Part model, mm, in its own coordinate system. Coordinates: 2 decimals unless noted, no trailing zeros. Loops run counter-clockwise (first coordinate to the right, second up) from the corner with the lowest first, then second, coordinate; pieces in that order, holes last. Notation, with made-up numbers: (-13.5, 50) - (-1.5, 50) arc R20 ccw to (-1.5, 54) - close; hole circle Ø9 at (82.25, 75). An arc over 180 degrees is marked (long way). Use a Markdown table: item, result. Add a question column.
1. Pull direction Z, two halves, no side cores. Call faces 1 (the flat face through (-4.5, 4, -2)), 2 (the cylindrical face through (0.66, 4.06, 0.43)): pulls with the +Z half, pulls with the -Z half, needs draft (parallel to the pull), parting line crosses it, or undercut.
2. Band-saw the part on D-D, the plane y = 3.25. Give the cut face in (x, z).
3. Band-saw the part on A-A, the plane z = 0. Give the cut face in (x, y).
4. Band-saw the part on B-B, the plane x = -1.25. Give the cut face in (y, z), plus the area to 3 significant figures.
5. Band-saw the part on C-C, the plane z = 5.25. Give the cut face in (x, y), plus the area to 3 significant figures.
6. Wall check: probe 1 along X at (y, z) = (6, -4.5); probe 2 along Y at (x, z) = (2.5, 0); probe 3 along Y at (x, z) = (1.5, 0.75). Give the ranges that are in metal, low to high. Write a range as [from, to].
7. Drop flat-ended pins along their axis: pin 1 (1.5 mm diameter, centred on y = 8, z = 0, fed in from -X); pin 2 (3 mm diameter, centred on x = 0.5, z = 4, fed in from -Y); pin 3 (3 mm diameter, centred on x = -1, z = 4.5, fed in from -Y); pin 4 (2 mm diameter, centred on x = -1, z = 3.5, fed in from +Y). Give the stop position or say it passes through.
from build123d import *

# Parameters (mm, degrees)
CUT_EXTRUDE2_OUTLINE_W = 3
CUT_EXTRUDE2_OUTLINE_H = 14.95468232
CUT_EXTRUDE2_DEPTH     = 12
HOLE1_D                = 4
HOLE1_DEPTH            = 12
HOLE1_CSINK_D          = 5
HOLE1_CSINK_ANGLE      = 45


with BuildPart() as part:
    # Sketch1 → Revolve1 (revolve)
    with BuildSketch(Plane.XY):
        with BuildLine():
            Line((0, 0), (0, 12))
            ThreePointArc((0, 12), (-6, 6), (0, 0))
        make_face()
    revolve(axis=Axis((0, 0, 0), (0, 1, 0)))

    # Cut-Extrude2: read off the stored shape, not the designer's step
    # Cut-Extrude2 outline → Cut-Extrude2 (cut)
    with BuildSketch(Plane(origin=(0, 0, 0), x_dir=(1, 0, 0), z_dir=(0, 1, 0))):
        with Locations((-6, 0)):
            Rectangle(CUT_EXTRUDE2_OUTLINE_W, CUT_EXTRUDE2_OUTLINE_H)
    cut_extrude2 = extrude(amount=CUT_EXTRUDE2_DEPTH, mode=Mode.SUBTRACT)

    # Mirror2: Cut-Extrude2 across plane
    add(cut_extrude2.mirror(Plane(origin=(0, 0, 0), x_dir=(0, 0, 1), z_dir=(1, 0, 0))), mode=Mode.SUBTRACT)

    # Hole1
    with Locations(Plane.ZY.offset(4.5)):
        with Locations((0, 6.01212861)):
            CounterSinkHole(HOLE1_D / 2, HOLE1_CSINK_D / 2, depth=HOLE1_DEPTH, counter_sink_angle=HOLE1_CSINK_ANGLE)


solid = part.part
Geometry check:
| question | item | result |
|---|---|---|
| 1 | face 1 | needs draft |
| 1 | face 2 | undercut |
| 2 | outline | (-4.5, -2.86) arc R5.33 ccw to (4.5, -2.86) - (4.5, 2.86) arc R5.33 ccw to (-4.5, 2.86) - close |
| 3 | outline | (-4.5, 2.03) arc R6 ccw to (4.5, 2.03) - (4.5, 4.01) - (-3.29, 4.01) - (-4.5, 3.51) - close; (-4.5, 8.51) - (-3.29, 8.01) - (4.5, 8.01) - (4.5, 9.97) arc R6 ccw to (-4.5, 9.97) - close |
| 4 | outline | circle Ø11.74 at (6, 0); hole circle Ø4 at (6.01, 0) |
| 4 | area | 95.6 mm^2 |
| 5 | outline | circle Ø5.81 at (0, 6) |
| 5 | area | 26.5 mm^2 |
| 6 | probe 1 | x = [-3.97, 3.97] |
| 6 | probe 2 | y = [0.55, 4.01], [8.01, 11.45] |
| 6 | probe 3 | y = [0.24, 4.16], [7.87, 11.76] |
| 7 | pin 1 | stops at x = -4.5 |
| 7 | pin 2 | stops at y = 0.56 |
| 7 | pin 3 | stops at y = 0.87 |
| 7 | pin 4 | stops at y = 11.39 |
